For this review, take the finished solid that the model builds, in its own axes (mm). A direction names the side the tool comes from. Give positions to 0.01 mm unless a question says otherwise; leave off trailing zeros. Write each loop counter-clockwise with the first axis right and the second up, starting at its lowest first coordinate (ties: lowest second). Pieces come first, ordered by that corner, then holes. Notation, with made-up numbers: (-4, 86) -> (1, 86) arc R30 cw to (1, 123) -> close; hole circle Ø6 at (76, 27). An arc over 180 degrees is marked (long way). Return JSON: item names as keys, results as strings.
from build123d import *

# Parameters (mm, degrees)
F1_DEPTH = 50.8
F2_T     = -6.35
F4_E4_W  = 76.2411638441
F4_E4_H  = 50.8
F5_DEPTH = 6.35
F4_E3_W  = 75.6305083632
F4_E3_H  = 50.8
F6_DEPTH = 6.35


# Not quite as in the source:
# - a feature of the source that left no trace in its solid (it failed there, or was rolled back) is left out
# - a pattern or mirror of a feature is missing from the dataset's text; its kind, count and spacing are read off the source's solid


with BuildPart() as f1:
    # F0 (on Top) → F1 (new body)
    with BuildSketch(Plane.XY):
        Polygon((76.1932209134, 0), (0, 76.1944577098), (-76.1932209134, 0), (-76.1932209134, -76.1944577098), (76.1932209134, -76.1944577098), align=None)
    extrude(amount=F1_DEPTH)

    # F2
    f2_openings = [f1.faces().sort_by_distance(p)[0] for p in [
        (0, -16.932102, 50.8),
    ]]
    offset(amount=F2_T, openings=f2_openings)

    # F4_E4 (on explicit) → F5 (join)
    with BuildSketch(Plane(origin=(75.6305083632, 76.2389451265, 0), x_dir=(0.0076290083, -0.9999708987, 0), z_dir=(-0.9999708987, -0.0076290083, 0))):
        with Locations((38.120581922, 25.4)):
            Rectangle(F4_E4_W, F4_E4_H)
    f5 = extrude(amount=F5_DEPTH)

    # F5_copies: F5 across plane
    add(f5.mirror(Plane(origin=(0, 0, 0), x_dir=(0, 0, -1), z_dir=(-1, 0, 0))))

    # F4_E3 (on explicit) → F6 (join)
    with BuildSketch(Plane.XZ.offset(-76.2389451265)):
        with Locations((37.8152541816, 25.4)):
            Rectangle(F4_E3_W, F4_E3_H)
    f6 = extrude(amount=F6_DEPTH)

    # F6_copies: F6 across plane
    add(f6.mirror(Plane(origin=(0, 0, 0), x_dir=(0, 0, -1), z_dir=(-1, 0, 0))))


solid = f1.part
1. For pin 1 (1.5 mm diameter, centred on x = -49.5, y = -35.5, fed in from +Z); pin 2 (1 mm diameter, centred on y = 10, z = 29, fed in from +X); pin 3 (1 mm diameter, centred on y = 60.5, z = 12.5, fed in from -X), all flat-tipped, find the tip position at first contact; note any pin that passes through.
Results found:
{"pin 1": "stops at z = 6.35", "pin 2": "stops at x = 76.14", "pin 3": "stops at x = -75.75"}
2. Add section C-C, the plane y = 13. State the section outline as (x, z) points, plus the area to 3 significant figures.
Results found:
{"outline": "(-76.11, 0) -> (-69.76, 0) -> (-69.76, 50.8) -> (-76.11, 50.8) -> close; (-63.19, 0) -> (63.19, 0) -> (63.19, 50.8) -> (54.21, 50.8) -> (54.21, 6.35) -> (-54.21, 6.35) -> (-54.21, 50.8) -> (-63.19, 50.8) -> close; (69.76, 0) -> (76.11, 0) -> (76.11, 50.8) -> (69.76, 50.8) -> close", "area": "2,250 mm²"}
3. Add section D-D, the plane y = -27.5. State the section outline as (x, z) points.
Results found:
{"outline": "(-76.19, 0) -> (76.19, 0) -> (76.19, 50.8) -> (69.84, 50.8) -> (69.84, 6.35) -> (-69.84, 6.35) -> (-69.84, 50.8) -> (-76.19, 50.8) -> close"}
4. Add section A-A, the plane z = 34.5. Count the separate pieces of the cut face and the enclosed holes in it, plus the area to 3 significant figures.
Results found:
{"separate pieces": "1", "enclosed holes": "3", "area": "4,920 mm²"}
5. To check wall thickness, follow probe 1 along X at (y, z) = (-3.5, 22); probe 2 along Y at (x, z) = (57, 15.5); probe 3 along Y at (x, z) = (28.5, 41). State the ranges of each line that lie inside material, in increasing order.
Results found:
{"probe 1": "x = -76.19 to -69.84, 69.84 to 76.19", "probe 2": "y = -76.19 to -69.84, 10.21 to 19.19, 69.89 to 76.24", "probe 3": "y = -76.19 to -69.84, 38.71 to 47.69, 69.89 to 76.24"}
6. Add section B-B, the plane x = -63. State the section outline as (y, z) points, plus the area to 3 significant figures.
Results found:
{"outline": "(-76.19, 0) -> (13.19, 0) -> (13.19, 50.8) -> (4.21, 50.8) -> (4.21, 6.35) -> (-69.84, 6.35) -> (-69.84, 50.8) -> (-76.19, 50.8) -> close; (69.89, 0) -> (76.24, 0) -> (76.24, 50.8) -> (69.89, 50.8) -> close", "area": "1,570 mm²"}
7. For faces 4 (the flat face through (-37, 69.889, 26)), 5 (the flat face through (-69.843, -36, 28)), 6 (the flat face through (76.193, -39, 25)), list the 3-axis set-ups (+Z, -Z, +X, -X, +Y, -Y) from which the entire face can be reached by the end or side of a thin tool; tool diameter is ignored.
Results found:
{"face 4": "+Z, -Z", "face 5": "+Z", "face 6": "+Z, -Z, +X, +Y, -Y"}
8. The part is to be moulded in two halves that separate along Y. For faces 1 (the flat face through (-34.433, 32.781, 28.264)), 2 (the flat face through (1, 76.239, 26)), 3 (the flat face through (29, 40, 50.8)), say which applies: +Y half, -Y half, draft (parallel to the pull), parting line (faces both ways), or undercut.
Results found:
{"face 1": "undercut", "face 2": "+Y half", "face 3": "draft"}
